CAD build for the part. Positions are in the model's coordinates, mm. A direction names the side the tool comes from. Coordinates: 2 decimals unless noted, no trailing zeros. Write each loop counter-clockwise with the first axis right and the second up, starting at its lowest first coordinate (ties: lowest second). Pieces come first, ordered by that corner, then holes. Notation, with made-up numbers: (-26.75, 55) -> (4.25, 55) arc R3 ccw to (4.25, 60) -> close; hole circle Ø3 at (26.5, 45.25). An arc over 180 degrees is marked (long way). Answer as CSV lines item,"result". Start each with the question number.
```python
from build123d import *

# Parameters (mm, degrees)
SKETCH1_R           = 3.5
BOSS_EXTRUDE1_DEPTH = 10
BOSS_EXTRUDE2_DEPTH = 4
SKETCH3_R           = 2
BOSS_EXTRUDE3_DEPTH = 2
SKETCH4_R           = 1.5
BOSS_EXTRUDE4_DEPTH = 1.5
SKETCH5_R           = 2
BOSS_EXTRUDE5_DEPTH = 5
SKETCH6_R           = 0.75
CUT_EXTRUDE1_DEPTH  = 5
SKETCH7_R           = 2.5
CUT_EXTRUDE2_DEPTH  = 8
SKETCH8_R           = 1.5
CUT_EXTRUDE4_DEPTH  = 5
SKETCH9_R           = 0.5
CUT_EXTRUDE5_DEPTH  = 15.056433877


with BuildPart() as part:
    # Sketch1 → Boss-Extrude1 (new body)
    with BuildSketch(Plane(origin=(0, 0, 0), x_dir=(1, 0, 0), z_dir=(0, 1, 0))):
        with Locations(Location((0, 0, 0), (0, 0, 270))):
            Circle(SKETCH1_R)
    extrude(amount=BOSS_EXTRUDE1_DEPTH)

    # Sketch2 → Boss-Extrude2 (add)
    with BuildSketch(Plane(origin=(0, 10, 0), x_dir=(1, 0, 0), z_dir=(0, 1, 0))):
        Polygon((2.020725942, 3.5), (-2.020725942, 3.5), (-4.041451884, 0), (-2.020725942, -3.5), (2.020725942, -3.5), (4.041451884, 0), align=None)
    extrude(amount=BOSS_EXTRUDE2_DEPTH)

    # Sketch3 → Boss-Extrude3 (add)
    with BuildSketch(Plane(origin=(0, 14, 0), x_dir=(1, 0, 0), z_dir=(0, 1, 0))):
        with Locations(Location((0, 0, 0), (0, 0, 270))):
            Circle(SKETCH3_R)
    extrude(amount=BOSS_EXTRUDE3_DEPTH)

    # Sketch4 → Boss-Extrude4 (add)
    with BuildSketch(Plane(origin=(0, 16, 0), x_dir=(1, 0, 0), z_dir=(0, 1, 0))):
        with Locations(Location((0, 0, 0), (0, 0, 270))):
            Circle(SKETCH4_R)
    extrude(amount=BOSS_EXTRUDE4_DEPTH)

    # Sketch5 → Boss-Extrude5 (add)
    with BuildSketch(Plane(origin=(0, 17.5, 0), x_dir=(1, 0, 0), z_dir=(0, 1, 0))):
        with Locations(Location((0, 0, 0), (0, 0, 270))):
            Circle(SKETCH5_R)
    extrude(amount=BOSS_EXTRUDE5_DEPTH)

    # Sketch6 → Cut-Extrude1 (cut)
    with BuildSketch(Plane(origin=(-1.299038106, 0, 0.75), x_dir=(0.5000000000000026, 0, 0.8660254037844373), z_dir=(-0.8660254037844373, 0, 0.5000000000000026))):
        with Locations(Location((0, 16.75, 0), (0, 0, 90))):
            Circle(SKETCH6_R)
    extrude(amount=-CUT_EXTRUDE1_DEPTH, mode=Mode.SUBTRACT)

    # Sketch7 → Cut-Extrude2 (cut)
    with BuildSketch(Plane.XZ):
        with Locations(Location((0, 0, 0), (0, 0, 270))):
            Circle(SKETCH7_R)
    extrude(amount=-CUT_EXTRUDE2_DEPTH, mode=Mode.SUBTRACT)

    # Sketch8 → Cut-Extrude4 (cut)
    with BuildSketch(Plane.XZ.offset(-8)):
        with Locations(Location((0, 0, 0), (0, 0, 270))):
            Circle(SKETCH8_R)
    extrude(amount=-CUT_EXTRUDE4_DEPTH, mode=Mode.SUBTRACT)

    # Sketch9 → Cut-Extrude5 (cut, through all)
    with BuildSketch(Plane.XZ.offset(-13)):
        with Locations(Location((0, 0, 0), (0, 0, 270))):
            Circle(SKETCH9_R)
    extrude(amount=-CUT_EXTRUDE5_DEPTH, mode=Mode.SUBTRACT)


solid = part.part
```
1. Cut at A-A (y = 12.75). Give the cut face in (x, z).
2. Cut at B-B (x = 3.25). Give the cut face in (y, z).
3. Mould opens along Z. For faces 1 (the face through (2, 14, -2)), 2 (the face through (0, 12, 3.5)), 3 (the face through (-0.488, 14.573, 0.108)) say: pulls with the +Z half, pulls with the -Z half, needs draft (parallel to the pull), parting line crosses it, or undercut.
4. Cut at D-D (y = 4.25). Give the cut face in (x, z).
5. Tool access for faces 4 (the face through (1.85, 10, -3.15)), 5 (the face through (-2, 15, 0)), 6 (the face through (0.45, 10.46, -1.43)): list every direction of +Z, -Z, +X, -X, +Y, -Y with a clear straight run to the whole face (end or side of a thin tool).
6. Flat gauge pins, fed straight in: P1, Ø1.5, axis at x = -0.5, z = -0.5, coming from the -Y side; P2, Ø1, axis at x = -3, y = 2.5, coming from the -Z side; P3, Ø1, axis at x = 1.5, y = 9, coming from the -Z side. Where does each tip first touch, or does it go through?
7. Cut at C-C (z = -3). Give the cut face in (x, y), then the cut area to 3 significant figures.
8. Wall check: line 1 (X direction, y = 14.15, z = 0); line 2 (X direction, y = 4.75, z = 0). Give the ranges that are in metal, low to high.
Geometry check:
1,outline,"(-4.04, 0) -> (-2.02, -3.5) -> (2.02, -3.5) -> (4.04, 0) -> (2.02, 3.5) -> (-2.02, 3.5) -> close; hole circle Ø3 at (0, 0)"
2,outline,"(0, -1.3) -> (10, -1.3) -> (10, -1.37) -> (14, -1.37) -> (14, 1.37) -> (10, 1.37) -> (10, 1.3) -> (0, 1.3) -> close"
3,face 1,"needs draft"
3,face 2,"pulls with the +Z half"
3,face 3,"undercut"
4,outline,"circle Ø7 at (0, 0); hole circle Ø5 at (0, 0)"
5,face 4,"-Z, +X, -Y"
5,face 5,"+Y"
5,face 6,"-Y"
6,P1,"y = 13"
6,P2,"z = -2.45"
6,P3,"z = -3.35"
7,outline,"(-2.31, 10) -> (-1.8, 10) -> (-1.8, 0) -> (1.8, 0) -> (1.8, 10) -> (2.31, 10) -> (2.31, 14) -> (-2.31, 14) -> close"
7,area,"54.5 mm²"
8,line 1,"-2 to -0.5, 0.5 to 2"
8,line 2,"-3.5 to -2.5, 2.5 to 3.5"
